```python
from build123d import *

# Parameters (mm, degrees)
SKETCH1_W            = 193
SKETCH1_H            = 53.1
BOSS_EXTRUDE1_DEPTH  = 6.8
SKETCH2_W            = 15
SKETCH2_H            = 6.8
BOSS_EXTRUDE2_DEPTH  = 6.8
SKETCH3_R            = 1.524
CUT_EXTRUDE1_DEPTH   = 6.8
FILLET1_R            = 3
FILLET1_OF_MIRROR1_R = 3


with BuildPart() as part:
    # Sketch1 → Boss-Extrude1 (new body)
    with BuildSketch(Plane.XY):
        Rectangle(SKETCH1_W, SKETCH1_H)
    extrude(amount=BOSS_EXTRUDE1_DEPTH)

    # Sketch2 → Boss-Extrude2 (add)
    with BuildSketch(Plane.XY.offset(6.8)):
        with Locations((0, 29.95)):
            Rectangle(SKETCH2_W, SKETCH2_H)
        with Locations((-71.5, 29.95)):
            Rectangle(SKETCH2_W, SKETCH2_H)
        with Locations((-71.5, -29.95)):
            Rectangle(SKETCH2_W, SKETCH2_H)
        with Locations((0, -29.95)):
            Rectangle(SKETCH2_W, SKETCH2_H)
    boss_extrude2 = extrude(amount=-BOSS_EXTRUDE2_DEPTH)

    # Sketch3 → Cut-Extrude1 (cut)
    with BuildSketch(Plane.XY.offset(6.8)):
        with Locations((-89, 0)):
            Circle(SKETCH3_R)
    cut_extrude1 = extrude(amount=-CUT_EXTRUDE1_DEPTH, mode=Mode.SUBTRACT)

    # Fillet1
    fillet1_edges = [part.edges().sort_by_distance(p)[0] for p in [
        (7.5, 33.35, 3.4),
        (-7.5, 33.35, 3.4),
        (-64, 33.35, 3.4),
        (-79, 33.35, 3.4),
        (7.5, -33.35, 3.4),
        (-7.5, -33.35, 3.4),
        (-64, -33.35, 3.4),
        (-79, -33.35, 3.4),
    ]]
    fillet(fillet1_edges, radius=FILLET1_R)

    # Mirror1: Boss-Extrude2, Cut-Extrude1 across plane
    add(boss_extrude2.mirror(Plane(origin=(0, 0, 0), x_dir=(0, 0, 1), z_dir=(1, 0, 0))))
    add(cut_extrude1.mirror(Plane(origin=(0, 0, 0), x_dir=(0, 0, 1), z_dir=(1, 0, 0))), mode=Mode.SUBTRACT)

    # Fillet1 of Mirror1
    fillet1_of_mirror1_edges = [part.edges().sort_by_distance(p)[0] for p in [
        (-7.5, 33.35, 3.4),
        (7.5, 33.35, 3.4),
        (64, 33.35, 3.4),
        (79, 33.35, 3.4),
        (-7.5, -33.35, 3.4),
        (7.5, -33.35, 3.4),
        (64, -33.35, 3.4),
        (79, -33.35, 3.4),
    ]]
    fillet(fillet1_of_mirror1_edges, radius=FILLET1_OF_MIRROR1_R)


solid = part.part
```
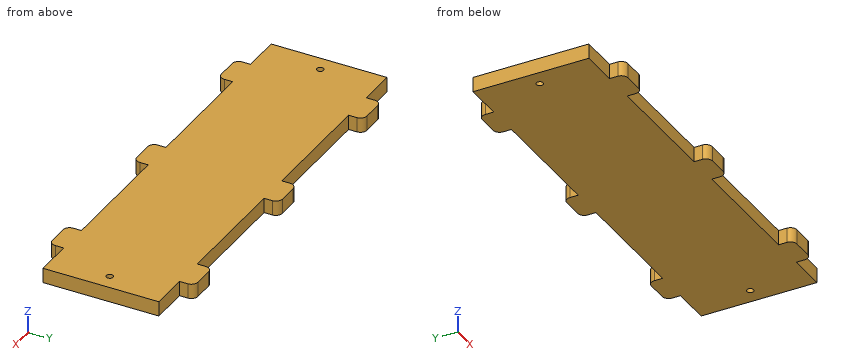
Input: part model. Units: mm. Frame: model coordinates. Coordinates: 2 decimals unless noted, no trailing zeros. Order: outer loops, then holes, each group sorted by start corner. A loop starts at its lowest first (then second) coordinate and runs counter-clockwise, first axis right, second up. Notation, with made-up numbers: (-15, 66.5) - (5, 66.5) arc R23 ccw to (5, 84.5) - close; hole circle Ø8 at (27.5, 30.5). An arc over 180 degrees is marked (long way). Put each result on its own line as item: value.
1. Cut plane A-A on z = 3.5. State how many separate pieces and enclosed holes the cut face has, then the cut area to 3 significant figures.
Report:
separate pieces: 1
enclosed holes: 2
area: 10,800 mm2
2. Cut plane B-B on x = 27.5. Return the cut outline in (y, z).
Report:
outline: (-26.55, 0) - (26.55, 0) - (26.55, 6.8) - (-26.55, 6.8) - close
3. Line query: line 1 along Y through (x, z) = (-89, 3); line 2 along X through (y, z) = (31.5, 2.5); line 3 along Y through (x, z) = (-20.5, 6.25). Output: solid intervals per line, ascending.
Report:
line 1: y = -26.55 to -1.52, 1.52 to 26.55
line 2: x = -78.77 to -64.23, -7.27 to 7.27, 64.23 to 78.77
line 3: y = -26.55 to 26.55
4. Contact query for flat-ended pins moving along their axis: pin 1 Ø1.9 at (y, z) = (28, 4) entering from -X; pin 2 Ø4 at (y, z) = (-28, 4.5) entering from +X; pin 3 Ø2 at (x, z) = (-41, 2) entering from +Y; pin 4 Ø2 at (x, z) = (86.5, 3) entering from -Y. Output: stop coordinate, or through.
Report:
pin 1: stops at x = -79
pin 2: stops at x = 96.5
pin 3: stops at y = 26.55
pin 4: stops at y = -26.55
